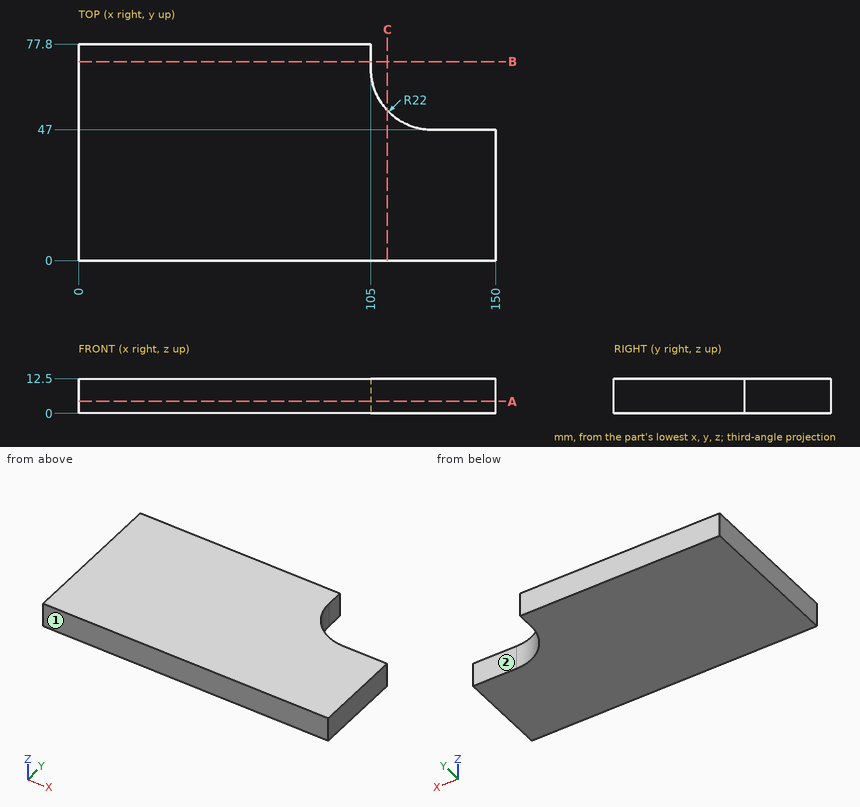
The drawing under review shows one solid part. Ordinate dimensions are in mm from its lowest x, y, z. A direction names the side the tool comes from. Round coordinates to 2 decimals unless told otherwise and drop trailing zeros. Write each loop counter-clockwise with the first axis right and the second up, starting at its lowest first coordinate (ties: lowest second). Pieces come first, ordered by that corner, then holes.
(1) We need section C-C on x = 111. Give the boundary of the cut face in (y, z), and give its area (3 significant figures).
(2) We need section B-B on y = 71.5. Give the boundary of the cut face in (x, z), and give its area (3 significant figures).
(3) Insertion check: pin 1 (1 mm diameter, centred on y = 67.5, z = 3.5, fed in from +X); pin 2 (4.5 mm diameter, centred on y = 75, z = 5, fed in from +X). Each pin has a flat end and moves straight along its axis. Give the tip position at first contact, or say it passes through.
(4) We need section A-A on z = 4.25. Give the boundary of the cut face in (x, y), and give its area (3 significant figures).
(5) Wall thickness on L1, parallel to X at y = 71, z = 6.75; L2, parallel to Y at x = 131, z = 10.5; L3, parallel to X at y = 56.5, z = 8: over which ranges is each line inside the solid? List them lowest first.
(6) Machinability: for the marked faces 1 and 2, which of the approach directions +Z, -Z, +X, -X, +Y, -Y give a long, thin tool a straight path to every point of the face, cutting with its end or side? Answer none if there is none.
Findings below:
1. outline: (0, 0) - (53.9, 0) - (53.9, 12.5) - (0, 12.5) - close
1. area: 674 mm2
2. outline: (0, 0) - (105, 0) - (105, 12.5) - (0, 12.5) - close
2. area: 1,310 mm2
3. pin 1: stops at x = 105.09
3. pin 2: stops at x = 105
4. outline: (0, 0) - (150, 0) - (150, 47) - (127, 47) arc R22 cw to (105, 69) - (105, 77.8) - (0, 77.8) - close
4. area: 10,400 mm2
5. L1: x = 0 to 105
5. L2: y = 0 to 47
5. L3: x = 0 to 108.9
6. face 1: +Z, -Z, +X, -X, -Y
6. face 2: +Z, -Z, +X, +Y
